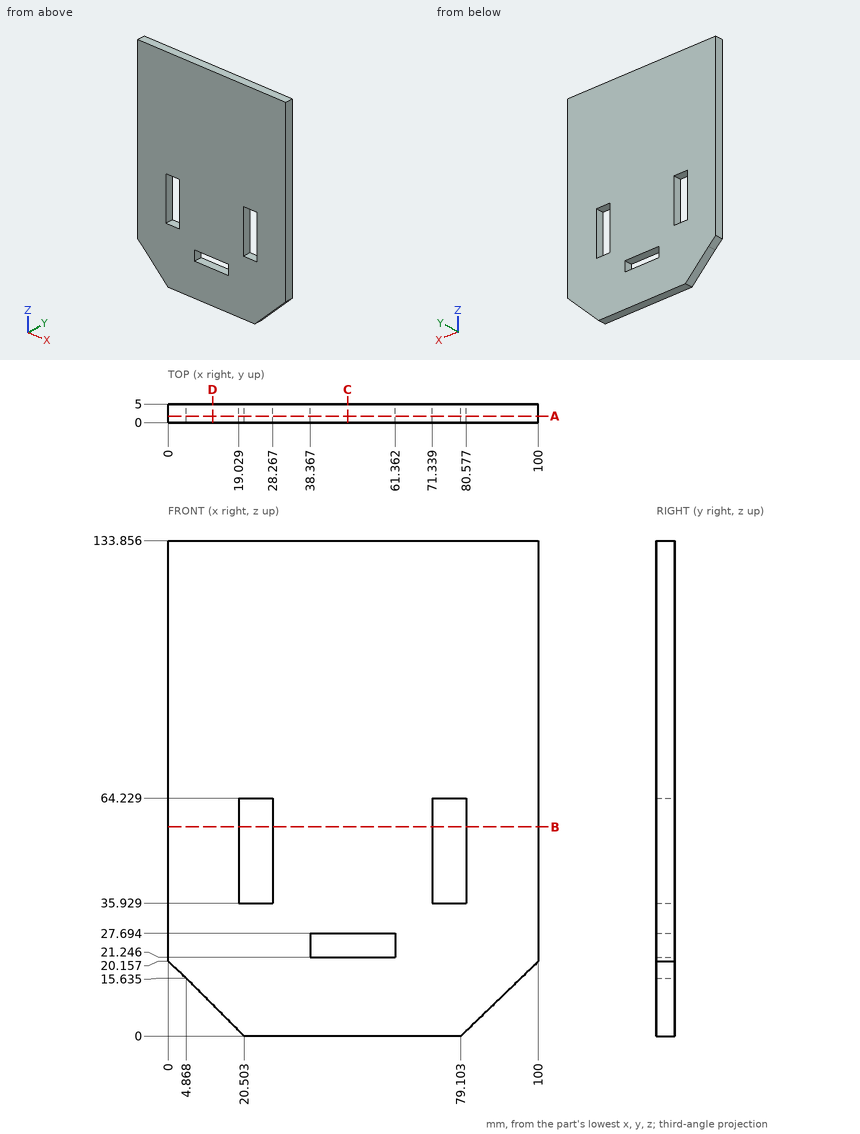
Drawing for the job (mm, zero at the part's lowest x, y, z). Give positions to 0.01 mm unless a question says otherwise; leave off trailing zeros. Write each loop counter-clockwise with the first axis right and the second up, starting at its lowest first coordinate (ties: lowest second). Pieces come first, ordered by that corner, then holes. Notation, with made-up numbers: (-12, 53.5) - (24, 53.5) arc R22 ccw to (24, 69.5) - close; hole circle Ø4 at (1, 21.25). An arc over 180 degrees is marked (long way). Answer as CSV lines item,"result".
Q1. Drill centre lines: line 1 (X direction, y = 4, z = 37.5); line 2 (Z direction, x = 24.5, y = 0.45) (1 decimal); line 3 (Z direction, x = 52, y = 3.2) (1 decimal). Where is each one in solid material? Low to high. Write a range as from..to.
Result set:
line 1,"0..19.03, 28.27..71.34, 80.58..100"
line 2,"0..35.9, 64.2..133.9"
line 3,"0..21.2, 27.7..133.9"
Q2. Band-saw the part on D-D (x = 12). Give the cut face in (y, z) (1 decimal), and give its area (3 significant figures).
Result set:
outline,"(0, 8.5) - (5, 8.5) - (5, 133.9) - (0, 133.9) - close"
area,"627 mm²"
Q3. Band-saw the part on A-A (y = 1.75). Give the cut face in (x, z) (1 decimal).
Result set:
outline,"(0, 20.2) - (4.9, 15.6) - (20.5, 0) - (79.1, 0) - (100, 20.2) - (100, 133.9) - (0, 133.9) - close; hole (19, 35.9) - (28.3, 35.9) - (28.3, 64.2) - (19, 64.2) - close; hole (38.4, 21.2) - (61.4, 21.2) - (61.4, 27.7) - (38.4, 27.7) - close; hole (71.3, 35.9) - (80.6, 35.9) - (80.6, 64.2) - (71.3, 64.2) - close"
Q4. Band-saw the part on C-C (x = 48.5). Give the cut face in (y, z) (1 decimal).
Result set:
outline,"(0, 0) - (5, 0) - (5, 21.2) - (0, 21.2) - close; (0, 27.7) - (5, 27.7) - (5, 133.9) - (0, 133.9) - close"
Q5. Flat gauge pin, fed straight in: pin 1 Ø1.5 at (y, z) = (4, 14.5) entering from +X. Where does the tip first touch, or does it go through?
Result set:
pin 1,"x = 94.91"
Q6. Band-saw the part on B-B (z = 56.5). Give the cut face in (x, y).
Result set:
outline,"(0, 0) - (19.03, 0) - (19.03, 5) - (0, 5) - close; (28.27, 0) - (71.34, 0) - (71.34, 5) - (28.27, 5) - close; (80.58, 0) - (100, 0) - (100, 5) - (80.58, 5) - close"
